The model under review builds one solid part; all positions refer to its coordinate system, in mm. Face numbers are marked on the shaded views. A direction names the side the tool comes from. Coordinates: 2 decimals unless noted, no trailing zeros. Order: outer loops, then holes, each group sorted by start corner. A loop starts at its lowest first (then second) coordinate and runs counter-clockwise, first axis right, second up. Notation, with made-up numbers: (78, 51) - (119, 51) arc R18 cw to (119, 77) - close; hole circle Ø10 at (2.25, -22.5). An arc over 180 degrees is marked (long way). Answer in a Markdown table with one row per item.
```python
from build123d import *

# Parameters (mm, degrees)
BOSS_EXTRUDE1_DEPTH = 12.7
CUT_EXTRUDE1_DEPTH  = 32.75


with BuildPart() as part:
    # Sketch1 → Boss-Extrude1 (new body)
    with BuildSketch(Plane(origin=(0, 0, 0), x_dir=(1, 0, 0), z_dir=(0, 1, 0))):
        Polygon((0, 0), (33.7947, 0), (33.7947, 1.5875), (33.7947, 31.75), (32.2072, 31.75), (32.2072, 1.5875), (1.5875, 1.5875), (1.5875, 11.176), (0, 11.176), (-31.75, 11.176), (-31.75, 9.5885), (0, 9.5885), (0, 1.5875), align=None)
    extrude(amount=BOSS_EXTRUDE1_DEPTH)

    # Sketch2 → Cut-Extrude1 (cut, through all)
    with BuildSketch(Plane.XY):
        with BuildLine():
            Line((5.3975, 7.90575), (11.7475, 7.90575))
            ThreePointArc((11.7475, 7.90575), (13.30325, 6.35), (11.7475, 4.79425))
            Line((11.7475, 4.79425), (5.3975, 4.79425))
            ThreePointArc((5.3975, 4.79425), (3.84175, 6.35), (5.3975, 7.90575))
        make_face()
        with BuildLine():
            Line((21.9075, 7.90575), (15.5575, 7.90575))
            ThreePointArc((15.5575, 7.90575), (14.00175, 6.35), (15.5575, 4.79425))
            Line((15.5575, 4.79425), (21.9075, 4.79425))
            ThreePointArc((21.9075, 4.79425), (23.46325, 6.35), (21.9075, 7.90575))
        make_face()
    extrude(amount=-CUT_EXTRUDE1_DEPTH, mode=Mode.SUBTRACT)


solid = part.part
```
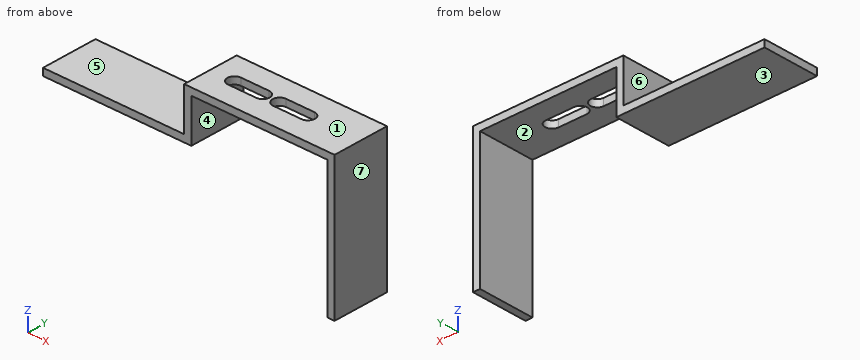
Item 1: We need section B-B, the plane x = 16.5. Write out the cut boundary in (y, z).
Check values:
| item | result |
|---|---|
| outline | (0, -1.59) - (4.79, -1.59) - (4.79, 0) - (0, 0) - close; (7.91, -1.59) - (12.7, -1.59) - (12.7, 0) - (7.91, 0) - close |
Item 2: To check wall thickness, follow line 1 (X direction, y = 11.5, z = -9); line 2 (Z direction, x = 16, y = 1.5); line 3 (X direction, y = 9.5, z = -22). State the ranges of each line that lie inside material, in increasing order. Write a range as from..to.
Check values:
| item | result |
|---|---|
| line 1 | 0..1.59, 32.21..33.79 |
| line 2 | -1.59..0 |
| line 3 | 32.21..33.79 |
Item 3: We need section C-C, the plane y = 11. Write out the cut boundary in (x, z), then the cut area to 3 significant figures.
Check values:
| item | result |
|---|---|
| outline | (-31.75, -11.18) - (1.59, -11.18) - (1.59, -1.59) - (32.21, -1.59) - (32.21, -31.75) - (33.79, -31.75) - (33.79, 0) - (0, 0) - (0, -9.59) - (-31.75, -9.59) - close |
| area | 167 mm^2 |
Item 4: We need section D-D, the plane x = -22.5. Write out the cut boundary in (y, z), then the cut area to 3 significant figures.
Check values:
| item | result |
|---|---|
| outline | (0, -11.18) - (12.7, -11.18) - (12.7, -9.59) - (0, -9.59) - close |
| area | 20.2 mm^2 |
Item 5: Clearance check with flat-ended pins moving along their axes: pin 1 Ø4 at (x, y) = (-7, 9) entering from -Z; pin 2 Ø3 at (x, z) = (2.5, -13.5) entering from -Y; pin 3 Ø6.5 at (y, z) = (3.5, -15.5) entering from -X; pin 4 Ø6.5 at (x, y) = (-10, 4) entering from +Z. State where each tip first meets the part, or that it passes through.
Check values:
| item | result |
|---|---|
| pin 1 | z = -11.18 |
| pin 2 | through |
| pin 3 | x = 32.21 |
| pin 4 | z = -9.59 |
Item 6: We need section A-A, the plane y = 6.35. Write out the cut boundary in (x, z).
Check values:
| item | result |
|---|---|
| outline | (-31.75, -11.18) - (1.59, -11.18) - (1.59, -1.59) - (3.84, -1.59) - (3.84, 0) - (0, 0) - (0, -9.59) - (-31.75, -9.59) - close; (13.3, -1.59) - (14, -1.59) - (14, 0) - (13.3, 0) - close; (23.46, -1.59) - (32.21, -1.59) - (32.21, -31.75) - (33.79, -31.75) - (33.79, 0) - (23.46, 0) - close |
Item 7: Mouldability with a two-part tool opening along X and no side actions: class the marked faces 4, 5, 6 and 7 as +X half, -X half, draft (parallel to the pull), parting line (faces both ways), or undercut.
Check values:
| item | result |
|---|---|
| face 4 | undercut |
| face 5 | draft |
| face 6 | -X half |
| face 7 | +X half |
Item 8: Tool access review of the marked faces 1, 2 and 3: name each direction out of +Z, -Z, +X, -X, +Y, -Y from which nothing blocks a thin tool from reaching the whole face with its end or side.
Check values:
| item | result |
|---|---|
| face 1 | +Z, +X, -X, +Y, -Y |
| face 2 | -Z, +Y, -Y |
| face 3 | -Z, -X, +Y, -Y |
